```python
from build123d import *

# Parameters (mm, degrees)
SKETCH004_W     = 40
SKETCH004_H     = 40
PAD001_DEPTH    = 35
FILLET001_R     = 5
SKETCH005_W     = 33
SKETCH005_H     = 33
POCKET003_DEPTH = 7
SKETCH006_W     = 5
SKETCH006_H     = 20
POCKET004_DEPTH = 2
SKETCH007_R     = 3.5
PAD002_DEPTH    = 4
SKETCH009_W     = 33
SKETCH009_H     = 33
POCKET006_DEPTH = 31
SKETCH010_W     = 14
SKETCH010_H     = 8
POCKET007_DEPTH = 4
SKETCH011_W     = 10.5
SKETCH011_H     = 6
POCKET008_DEPTH = 4
PAD003_DEPTH    = 2
SKETCH013_R     = 1.5
POCKET009_DEPTH = 8
POCKET010_DEPTH = 2
PAD004_DEPTH    = 0.4


with BuildPart() as part:
    # Sketch004 → Pad001 (new body)
    with BuildSketch(Plane.XY):
        Rectangle(SKETCH004_W, SKETCH004_H)
    extrude(amount=PAD001_DEPTH)

    # Fillet001
    fillet001_edges = [part.edges().sort_by_distance(p)[0] for p in [
        (-20, -20, 17.5),
        (20, -20, 17.5),
        (20, 20, 17.5),
        (-20, 20, 17.5),
    ]]
    fillet(fillet001_edges, radius=FILLET001_R)

    # Sketch005 (on Face2 of Fillet001) → Pocket003 (cut)
    with BuildSketch(Plane(origin=(0, 0, 0), x_dir=(1, 0, 0), z_dir=(0, 0, -1))):
        Rectangle(SKETCH005_W, SKETCH005_H)
    extrude(amount=-POCKET003_DEPTH, mode=Mode.SUBTRACT)

    # Sketch006 (on Face15 of Pocket003) → Pocket004 (cut)
    with BuildSketch(Plane(origin=(0, 0, 7), x_dir=(1, 0, 0), z_dir=(0, 0, -1))):
        with Locations((13, 4)):
            Rectangle(SKETCH006_W, SKETCH006_H)
    extrude(amount=-POCKET004_DEPTH, mode=Mode.SUBTRACT)

    # Sketch007 (on Face15 of Pocket004) → Pad002 (join)
    with BuildSketch(Plane(origin=(0, 0, 7), x_dir=(1, 0, 0), z_dir=(0, 0, -1))):
        with Locations((-11, 11)):
            Circle(SKETCH007_R)
        with Locations((11, -11)):
            Circle(SKETCH007_R)
    extrude(amount=PAD002_DEPTH)

    # Sketch009 → Pocket006 (cut)
    with BuildSketch(Plane.XY.offset(40)):
        Rectangle(SKETCH009_W, SKETCH009_H)
    extrude(amount=-POCKET006_DEPTH, mode=Mode.SUBTRACT)

    # Sketch010 (on Face14 of Pocket006) → Pocket007 (cut)
    with BuildSketch(Plane.XZ.offset(-16.5)):
        with Locations((-6.75, 5.5)):
            Rectangle(SKETCH010_W, SKETCH010_H)
    extrude(amount=-POCKET007_DEPTH, mode=Mode.SUBTRACT)

    # Sketch011 (on Face17 of Pocket007) → Pocket008 (cut)
    with BuildSketch(Plane.XZ.offset(-16.5)):
        with Locations((-7.49469, 18.159044)):
            Rectangle(SKETCH011_W, SKETCH011_H)
    extrude(amount=-POCKET008_DEPTH, mode=Mode.SUBTRACT)

    # Sketch012 (on Face28 of Pocket008) → Pad003 (join)
    with BuildSketch(Plane.XY.offset(9)):
        with BuildLine():
            Line((16.5, 16.5), (6.5, 16.5))
            Line((6.5, 16.5), (6.5, 10.808341))
            ThreePointArc((6.5, 10.808341), (7.815135, 7.815135), (10.808341, 6.5))
            Line((10.808341, 6.5), (16.5, 6.5))
            Line((16.5, 6.5), (16.5, 16.5))
        make_face()
        with BuildLine():
            Line((-16.5, -16.5), (-6.5, -16.5))
            Line((-6.5, -16.5), (-6.5, -10.808341))
            ThreePointArc((-6.5, -10.808341), (-7.815135, -7.815135), (-10.808341, -6.5))
            Line((-10.808341, -6.5), (-16.5, -6.5))
            Line((-16.5, -6.5), (-16.5, -16.5))
        make_face()
    extrude(amount=PAD003_DEPTH)

    # Sketch013 (on Face45 of Pad003) → Pocket009 (cut)
    with BuildSketch(Plane(origin=(0, 0, 3), x_dir=(1, 0, 0), z_dir=(0, 0, -1))):
        with Locations((-11, 11)):
            Circle(SKETCH013_R)
        with Locations((11, -11)):
            Circle(SKETCH013_R)
    extrude(amount=-POCKET009_DEPTH, mode=Mode.SUBTRACT)

    # Sketch014 (on Face30 of Pocket009) → Pocket010 (cut)
    with BuildSketch(Plane.XY.offset(11)):
        Polygon((13.6, 11), (12.3, 13.251666), (9.7, 13.251666), (8.4, 11), (9.7, 8.748334), (12.3, 8.748334), align=None)
        Polygon((-8.4, -11), (-9.7, -8.748334), (-12.3, -8.748334), (-13.6, -11), (-12.3, -13.251666), (-9.7, -13.251666), align=None)
    extrude(amount=-POCKET010_DEPTH, mode=Mode.SUBTRACT)

    # Sketch015 (on Face27 of Pocket010) → Pad004 (join)
    with BuildSketch(Plane(origin=(0, 0, 7), x_dir=(1, 0, 0), z_dir=(0, 0, -1))):
        Polygon((-16.5, 16.5), (16.5, 16.5), (16.5, -16.5), (0.25, -16.5), (0.25, -13.5), (6, -13.5), (6, -6), (15.5, -6), (15.5, 14), (-6.25, 14), (-6.25, 6.5), (-13.75, 6.5), (-13.75, -16.5), (-16.5, -16.5), align=None)
    extrude(amount=PAD004_DEPTH)


with BuildPart() as part_1:
    # Body001 placement: moved
    add(part.part.moved(Location((0, 0, 3))))


solid = part_1.part
```
The listing builds one solid part. Answer for the finished solid, in the listing's coordinates (mm). A direction names the side the tool comes from. Give positions to 0.01 mm unless a question says otherwise; leave off trailing zeros. Order: outer loops, then holes, each group sorted by start corner. A loop starts at its lowest first (then second) coordinate and runs counter-clockwise, first axis right, second up. Notation, with made-up numbers: (32.5, 7.5) - (89.5, 7.5) arc R20 cw to (89.5, 45.5) - close; hole circle Ø1 at (65, 41). An arc over 180 degrees is marked (long way). Use one line per item in the form item = value. Start each with the question number.
(1) For faces 1 (the flat face through (-9.06, -12.14, 13.01)), 2 (the flat face through (-18, 0, 3)), 3 (the flat face through (-8, -7, 9.6)), determine the directions among +Z, -Z, +X, -X, +Y, -Y from which every point of the face is accessible in a straight line to the end or side of a thin tool.
(2) A cutting plane is placed at C-C, the plane z = 27. Write down the section's boundary in (x, y), then the cut area to 3 significant figures.
(3) The mould has two halves that part along Y. Classify faces 4 (the flat face through (0.25, 18, 9)), 5 (the flat face through (-11, -11, 10)), 6 (the cylindrical face through (18, -19, 21)): released by +Y, released by -Y, zero draft, split by the parting line, or undercut.
(4) Flat-ended cylindrical pins translate along their axes: pin 1 Ø1 at (y, z) = (19, 20.5) entering from -X; pin 2 Ø10 at (x, y) = (-4, 3) entering from +Z; pin 3 Ø1 at (x, y) = (9.5, -9.5) entering from -Z. Find the tip coordinate at first contact, or state that the pin passes through.
(5) A cutting plane is placed at A-A, the plane x = -4.5. Write down the section's boundary in (y, z), then the cut area to 3 significant figures.
(6) Consider line 1 (Y direction, x = -11, z = 7.9); line 2 (X direction, y = -11, z = 11.2); line 3 (X direction, y = -11, z = 8.25). Determine where each line is inside the solid, lowest interval first. Write a range as from..to.
(7) A cutting plane is placed at D-D, the plane x = 5. Write down the section's boundary in (y, z), then the cut area to 3 significant figures.
Ans:
q1.face_1 = +Z
q1.face_2 = -Z, +X, -X, +Y, -Y
q1.face_3 = -Z
q2.outline = (-20, -15) arc R5 ccw to (-15, -20) - (15, -20) arc R5 ccw to (20, -15) - (20, 15) arc R5 ccw to (15, 20) - (-15, 20) arc R5 ccw to (-20, 15) - close; hole (-16.5, -16.5) - (16.5, -16.5) - (16.5, 16.5) - (-16.5, 16.5) - close
q2.area = 490 mm^2
q3.face_4 = zero draft
q3.face_5 = undercut
q3.face_6 = released by -Y
q4.pin_1 = -18.57
q4.pin_2 = 12
q4.pin_3 = 10
q5.outline = (-20, 3) - (-16.5, 3) - (-16.5, 9.6) - (-14, 9.6) - (-14, 10) - (16.5, 10) - (16.5, 12) - (-16.5, 12) - (-16.5, 38) - (-20, 38) - close; (16.5, 3) - (20, 3) - (20, 4.5) - (16.5, 4.5) - close; (16.5, 12.5) - (20, 12.5) - (20, 18.16) - (16.5, 18.16) - close; (16.5, 24.16) - (20, 24.16) - (20, 38) - (16.5, 38) - close
q5.area = 263 mm^2
q6.line_1 = -20..-16.5, -14.5..-12.5, -9.5..-7.5
q6.line_2 = -20..-12.5, -9.5..10.5, 15.5..20
q6.line_3 = -20..-16.5, -14.5..-12.5, -9.5..-7.5, 16.5..20
q7.outline = (-20, 3) - (-16.5, 3) - (-16.5, 9.6) - (-14, 9.6) - (-14, 10) - (13.5, 10) - (13.5, 9.6) - (16.5, 9.6) - (16.5, 3) - (20, 3) - (20, 38) - (16.5, 38) - (16.5, 12) - (-16.5, 12) - (-16.5, 38) - (-20, 38) - close
q7.area = 313 mm^2
